from build123d import *

# Parameters (mm, degrees)
SKETCH1_R               = 12.9
SKETCH1_R_2             = 8.1
BOSS_EXTRUDE1_DEPTH     = 8
CUT_EXTRUDE1_DEPTH      = 1
CUT_EXTRUDE1_DEPTH_BACK = 1
SKETCH3_R               = 8.805307923
SKETCH4_R               = 1
CUT_EXTRUDE2_DEPTH      = 6
FILLET1_R               = 3
FILLET2_R               = 5
SKETCH5_R               = 1
CUT_EXTRUDE3_DEPTH      = 10
DRAFT4_ANGLE            = -10
DRAFT6_ANGLE            = -10
SKETCH6_R               = 1
CUT_EXTRUDE4_DEPTH      = 10
BOSS_EXTRUDE3_START     = 1
SKETCH7_R               = 8.1
BOSS_EXTRUDE3_DEPTH     = 1
SKETCH11_R              = 8.1
BOSS_EXTRUDE4_DEPTH     = 1
SKETCH12_OUTSIDE_W      = 157.242
SKETCH12_OUTSIDE_H      = 107.242
SKETCH12_OUTSIDE_R      = 12.9
CUT_EXTRUDE5_DEPTH      = 108.3070569


with BuildPart() as part:
    # Sketch1 → Boss-Extrude1 (new body)
    # profile 1 of 8: a face of its own
    with BuildSketch(Plane.XY):
        with Locations((-26.538003558, 0)):
            Circle(SKETCH1_R)
        with Locations((-26.538003558, 0)):
            Circle(SKETCH1_R_2, mode=Mode.SUBTRACT)
    # profile 2 of 8: a face of its own
    with BuildSketch(Plane.XY):
        with BuildLine():
            ThreePointArc((-21.664910941, 11.944160429), (-17.46502072, 9.170113544), (-14.646409889, 5))
            Line((-14.646409889, 5), (-14.466935746, 5))
            Line((-14.466935746, 5), (18.588903825, 38.055839571))
            ThreePointArc((18.588903825, 38.055839571), (14.340318965, 40.878322523), (11.517836013, 45.126907383))
            Line((11.517836013, 45.126907383), (-21.664910941, 11.944160429))
        make_face()
    # profile 3 of 8: a face of its own
    with BuildSketch(Plane.XY):
        with BuildLine():
            Line((-14.466935746, 5), (-14.646409889, 5))
            ThreePointArc((-14.646409889, 5), (-14.619957589, 4.936616278), (-14.593843129, 4.873092617))
            Line((-14.593843129, 4.873092617), (-14.466935746, 5))
        make_face()
    # profile 4 of 8: a face of its own
    with BuildSketch(Plane.XY):
        with BuildLine():
            Line((61.39092863, 5), (-14.466935746, 5))
            Line((-14.466935746, 5), (-14.593843129, 4.873092617))
            ThreePointArc((-14.593843129, 4.873092617), (-13.879218673, 2.482975077), (-13.638003558, 0))
            ThreePointArc((-13.638003558, 0), (-13.892617871, -2.550337396), (-14.646409889, -5))
            Line((-14.646409889, -5), (61.570402773, -5))
            ThreePointArc((61.570402773, -5), (60.56217928, -0.068681781), (61.517836013, 4.873092617))
            Line((61.517836013, 4.873092617), (61.39092863, 5))
        make_face()
    # profile 5 of 8: a face of its own
    with BuildSketch(Plane.XY):
        with Locations((23.461996442, 50)):
            Circle(SKETCH1_R)
        with Locations((23.461996442, 50)):
            Circle(SKETCH1_R_2, mode=Mode.SUBTRACT)
    # profile 6 of 8: a face of its own
    with BuildSketch(Plane.XY):
        with BuildLine():
            Line((28.335089059, 38.055839571), (61.39092863, 5))
            Line((61.39092863, 5), (61.570402773, 5))
            ThreePointArc((61.570402773, 5), (64.389013604, 9.170113544), (68.588903825, 11.944160429))
            Line((68.588903825, 11.944160429), (35.406156871, 45.126907383))
            ThreePointArc((35.406156871, 45.126907383), (32.583673919, 40.878322523), (28.335089059, 38.055839571))
        make_face()
    # profile 7 of 8: a face of its own
    with BuildSketch(Plane.XY):
        with Locations((73.461996442, 0)):
            Circle(SKETCH1_R)
        with Locations((73.461996442, 0)):
            Circle(SKETCH1_R_2, mode=Mode.SUBTRACT)
    # profile 8 of 8: a face of its own
    with BuildSketch(Plane.XY):
        with BuildLine():
            Line((61.570402773, 5), (61.39092863, 5))
            Line((61.39092863, 5), (61.517836013, 4.873092617))
            ThreePointArc((61.517836013, 4.873092617), (61.543950473, 4.936616278), (61.570402773, 5))
        make_face()
    extrude(amount=BOSS_EXTRUDE1_DEPTH)

    # Sketch3 → Cut-Extrude1 (cut, two sides: drawn at the far end of the back side and taken through both)
    with BuildSketch(Plane.XY.offset(4).offset(-CUT_EXTRUDE1_DEPTH_BACK)):
        with Locations((-26.538003558, 0)):
            Circle(SKETCH3_R)
        with Locations((23.461996442, 50)):
            Circle(SKETCH3_R)
        with Locations((73.461996442, 0)):
            Circle(SKETCH3_R)
    extrude(amount=CUT_EXTRUDE1_DEPTH + CUT_EXTRUDE1_DEPTH_BACK, mode=Mode.SUBTRACT)

    # Sketch4 → Cut-Extrude2 (cut)
    with BuildSketch(Plane(origin=(0, 63.1, 0), x_dir=(-1, 0, 0), z_dir=(0, -1, 0))):
        with Locations(Location((-23.511996442, -4, 0), (0, 0, 270))):
            Circle(SKETCH4_R)
    extrude(amount=CUT_EXTRUDE2_DEPTH, mode=Mode.SUBTRACT)

    # Fillet1
    fillet1_edges = [part.edges().sort_by_distance(p)[0] for p in [
        (61.39092863, 5, 4),
        (28.335089059, 38.055839571, 4),
        (18.588903825, 38.055839571, 4),
        (-14.466935746, 5, 4),
    ]]
    fillet(fillet1_edges, radius=FILLET1_R)

    # Fillet2
    fillet2_edges = [part.edges().sort_by_distance(p)[0] for p in [
        (68.588903825, 11.944160429, 4),
        (61.570402773, -5, 4),
        (-14.646409889, -5, 4),
        (-21.664910941, 11.944160429, 4),
        (11.517836013, 45.126907383, 4),
        (35.406156871, 45.126907383, 4),
    ]]
    fillet(fillet2_edges, radius=FILLET2_R)

    # Sketch5 → Cut-Extrude3 (cut)
    with BuildSketch(Plane(origin=(45.994097055, -45.994097055, 0), x_dir=(0, 0, 1), z_dir=(-0.7071067811865489, 0.7071067811865462, 0))):
        with Locations(Location((4, 51.995475844, 0), (0, 0, 90))):
            Circle(SKETCH5_R)
    extrude(amount=CUT_EXTRUDE3_DEPTH, mode=Mode.SUBTRACT)

    # Draft4
    draft4_faces = [part.faces().sort_by_distance(p)[0] for p in [
        (-34.638003558, 0, 6.5),
        (15.361996442, 50, 6.5),
        (65.361996442, 0, 6.5),
    ]]
    draft(draft4_faces, Plane.XY.offset(8), DRAFT4_ANGLE)

    # Draft6
    draft6_faces = [part.faces().sort_by_distance(p)[0] for p in [
        (-34.638003558, 0, 1.5),
        (65.361996442, 0, 1.5),
        (15.361996442, 50, 1.5),
    ]]
    draft(draft6_faces, Plane(origin=(0, 0, 0), x_dir=(-1, 0, 0), z_dir=(0, 0, -1)), DRAFT6_ANGLE)

    # Sketch6 → Cut-Extrude4 (cut)
    with BuildSketch(Plane(origin=(-22.532100613, -22.532100613, 0), x_dir=(0, 0, -1), z_dir=(0.7071067811865486, 0.7071067811865465, 0))):
        with Locations(Location((-4, 18.715202275, 0), (0, 0, 270))):
            Circle(SKETCH6_R)
    extrude(amount=CUT_EXTRUDE4_DEPTH, mode=Mode.SUBTRACT)

    # Sketch7 → Boss-Extrude3 (add)
    with BuildSketch(Plane.XY.offset(8).offset(BOSS_EXTRUDE3_START)):
        with BuildLine():
            Line((66.499673424, 14.03339083), (37.495387272, 43.037676982))
            ThreePointArc((37.495387272, 43.037676982), (36.248927219, 45.112891138), (36.123400302, 47.53041455))
            ThreePointArc((36.123400302, 47.53041455), (23.461996442, 62.9), (10.800592582, 47.53041455))
            ThreePointArc((10.800592582, 47.53041455), (10.675065665, 45.112891138), (9.428605612, 43.037676982))
            Line((9.428605612, 43.037676982), (-19.57568054, 14.03339083))
            ThreePointArc((-19.57568054, 14.03339083), (-21.650894696, 12.786930777), (-24.068418108, 12.66140386))
            ThreePointArc((-24.068418108, 12.66140386), (-38.456049527, -4.936616278), (-15.838778411, -7.206703911))
            ThreePointArc((-15.838778411, -7.206703911), (-14.040570278, -5.586017646), (-11.69179192, -5))
            Line((-11.69179192, -5), (58.615784804, -5))
            ThreePointArc((58.615784804, -5), (60.964563162, -5.586017646), (62.762771295, -7.206703911))
            ThreePointArc((62.762771295, -7.206703911), (85.380042411, -4.936616278), (70.992410992, 12.66140386))
            ThreePointArc((70.992410992, 12.66140386), (68.57488758, 12.786930777), (66.499673424, 14.03339083))
        make_face()
        with Locations((-26.538003558, 0)):
            Circle(SKETCH7_R, mode=Mode.SUBTRACT)
        with Locations((73.461996442, 0)):
            Circle(SKETCH7_R, mode=Mode.SUBTRACT)
        with Locations((23.461996442, 50)):
            Circle(SKETCH7_R, mode=Mode.SUBTRACT)
        with BuildLine():
            Line((-7.224295059, 5), (54.148287943, 5))
            ThreePointArc((54.148287943, 5), (56.919926541, 6.851949703), (56.269608287, 10.121320344))
            Line((56.269608287, 10.121320344), (29.642686082, 36.748242548))
            ThreePointArc((29.642686082, 36.748242548), (28.303088236, 37.523283704), (26.755447003, 37.52750292))
            ThreePointArc((26.755447003, 37.52750292), (23.461996442, 37.1), (20.168545881, 37.52750292))
            ThreePointArc((20.168545881, 37.52750292), (18.620904648, 37.523283704), (17.281306802, 36.748242548))
            Line((17.281306802, 36.748242548), (-9.345615403, 10.121320344))
            ThreePointArc((-9.345615403, 10.121320344), (-9.995933657, 6.851949703), (-7.224295059, 5))
        make_face(mode=Mode.SUBTRACT)
    extrude(amount=-BOSS_EXTRUDE3_DEPTH)

    # Sketch11 → Boss-Extrude4 (add)
    with BuildSketch(Plane(origin=(0, 0, 0), x_dir=(-1, 0, 0), z_dir=(0, 0, -1))):
        with BuildLine():
            Line((-37.495387272, 43.037676982), (-66.499673424, 14.03339083))
            ThreePointArc((-66.499673424, 14.03339083), (-68.57488758, 12.786930777), (-70.992410992, 12.66140386))
            ThreePointArc((-70.992410992, 12.66140386), (-85.380042411, -4.936616278), (-62.762771295, -7.206703911))
            ThreePointArc((-62.762771295, -7.206703911), (-60.964563162, -5.586017646), (-58.615784804, -5))
            Line((-58.615784804, -5), (11.69179192, -5))
            ThreePointArc((11.69179192, -5), (14.040570278, -5.586017646), (15.838778411, -7.206703911))
            ThreePointArc((15.838778411, -7.206703911), (38.456049527, -4.936616278), (24.068418108, 12.66140386))
            ThreePointArc((24.068418108, 12.66140386), (21.650894696, 12.786930777), (19.57568054, 14.03339083))
            Line((19.57568054, 14.03339083), (-9.428605612, 43.037676982))
            ThreePointArc((-9.428605612, 43.037676982), (-10.675065665, 45.112891138), (-10.800592582, 47.53041455))
            ThreePointArc((-10.800592582, 47.53041455), (-23.461996442, 62.9), (-36.123400302, 47.53041455))
            ThreePointArc((-36.123400302, 47.53041455), (-36.248927219, 45.112891138), (-37.495387272, 43.037676982))
        make_face()
        with Locations(Location((-73.461996442, 0, 0), (0, 0, 180))):
            Circle(SKETCH11_R, mode=Mode.SUBTRACT)
        with Locations(Location((-23.461996442, 50, 0), (0, 0, 180))):
            Circle(SKETCH11_R, mode=Mode.SUBTRACT)
        with Locations(Location((26.538003558, 0, 0), (0, 0, 180))):
            Circle(SKETCH11_R, mode=Mode.SUBTRACT)
        with BuildLine():
            Line((-17.281306802, 36.748242548), (9.345615403, 10.121320344))
            ThreePointArc((9.345615403, 10.121320344), (9.995933657, 6.851949703), (7.224295059, 5))
            Line((7.224295059, 5), (-54.148287943, 5))
            ThreePointArc((-54.148287943, 5), (-56.919926541, 6.851949703), (-56.269608287, 10.121320344))
            Line((-56.269608287, 10.121320344), (-29.642686082, 36.748242548))
            ThreePointArc((-29.642686082, 36.748242548), (-28.303088236, 37.523283704), (-26.755447003, 37.52750292))
            ThreePointArc((-26.755447003, 37.52750292), (-23.461996442, 37.1), (-20.168545881, 37.52750292))
            ThreePointArc((-20.168545881, 37.52750292), (-18.620904648, 37.523283704), (-17.281306802, 36.748242548))
        make_face(mode=Mode.SUBTRACT)
    extrude(amount=BOSS_EXTRUDE4_DEPTH)

    # Sketch12 outside → Cut-Extrude5 (cut, through all)
    with BuildSketch(Plane(origin=(0, 0, -1), x_dir=(-1, 0, 0), z_dir=(0, 0, -1))):
        with Locations((-23.462, 25)):
            Rectangle(SKETCH12_OUTSIDE_W, SKETCH12_OUTSIDE_H)
        with Locations((-73.461996442, 0)):
            Circle(SKETCH12_OUTSIDE_R, mode=Mode.SUBTRACT)
    extrude(amount=-CUT_EXTRUDE5_DEPTH, mode=Mode.SUBTRACT)


solid = part.part
Input: part model. Units: mm. Frame: model coordinates. A direction names the side the tool comes from. Coordinates: 2 decimals unless noted, no trailing zeros. Loops run counter-clockwise (first coordinate to the right, second up) from the corner with the lowest first, then second, coordinate; pieces in that order, holes last. Notation, with made-up numbers: (28.25, 11.5) - (68.25, 11.5) arc R30 cw to (68.25, 41.5) - close; hole circle Ø8 at (-17.5, -22.75). An arc over 180 degrees is marked (long way). Answer in a Markdown table with one row per item. Add a question column.
Item 1: Section query A-A on y = 0. Return the cut outline in (x, z).
Item 2: Mould query, pull axis X, two halves, no side actions, for faces 1 (the conical face through (80.975, -3.115, 7.812)), 2 (the flat face through (82, 0, 9)). Classes: released by +X, released by -X, zero draft, split by the parting line, or undercut.
Item 3: Contact query for flat-ended pins moving along their axis: P1, Ø3, axis at x = 79, z = 3, coming from the -Y side; P2, Ø6, axis at x = 68, z = 0, coming from the +Y side; P3, Ø1, axis at y = 10, z = 8, coming from the -X side (3 decimals); P4, Ø14, axis at x = 69, y = -4.5, coming from the -Z side. Output: stop coordinate, or through.
Item 4: Access query for faces 3 (the cylindrical face through (65.37, 0.36, 8.51)), 4 (the conical face through (80.97, -3.11, 0.15)). Directions: +Z, -Z, +X, -X, +Y, -Y. A direction counts if a zero-diameter tool reaches every point of the face in a straight line with its end or side. Return the directions, or none.
Item 5: Section query C-C on z = 7. Return the cut outline in (x, y).
Item 6: Line query: line 1 along X through (y, z) = (0, 4.1); line 2 along Z through (x, y) = (65, -2); line 3 along X through (y, z) = (2.25, 8.25). Output: solid intervals per line, ascending. Write a range as [from, to].
Item 7: Section query B-B on z = 0.5. Return the cut outline in (x, y).
Recorded:
| question | item | result |
|---|---|---|
| 1 | outline | (60.56, -1) - (65.36, -1) - (65.36, 0) - (64.83, 3) - (64.66, 3) - (64.66, 5) - (64.83, 5) - (65.36, 8) - (65.36, 9) - (60.56, 9) - close; (81.56, -1) - (86.36, -1) - (86.36, 9) - (81.56, 9) - (81.56, 8) - (82.09, 5) - (82.27, 5) - (82.27, 3) - (82.09, 3) - (81.56, 0) - close |
| 2 | face 1 | undercut |
| 2 | face 2 | zero draft |
| 3 | P1 | y = -12.25 |
| 3 | P2 | y = 12.66 |
| 3 | P3 | x = 64.735 |
| 3 | P4 | z = -1 |
| 4 | face 3 | +Z, -Z |
| 4 | face 4 | none |
| 5 | outline | circle Ø25.8 at (73.46, 0); hole circle Ø16.55 at (73.46, 0) |
| 6 | line 1 | [60.56, 64.66], [82.27, 86.36] |
| 6 | line 2 | [-1, 3], [5, 9] |
| 6 | line 3 | [60.76, 65.68], [81.24, 86.16] |
| 7 | outline | circle Ø25.8 at (73.46, 0); hole circle Ø16.38 at (73.46, 0) |
